Can you work these out from the model? Positions are in its coordinate system, mm. A direction names the side the tool comes from. Give positions to 0.01 mm unless a question says otherwise; leave off trailing zeros. Order: outer loops, then holes, each group sorted by start corner. A loop starts at its lowest first (then second) coordinate and runs counter-clockwise, first axis right, second up. Notation, with made-up numbers: (59, 72) - (74, 72) arc R24 ccw to (74, 109) - close; hole circle Ø9 at (50.25, 35.25). An arc over 180 degrees is marked (long way). Use one line per item in the form item = value. Start each with the question number.
1) Suppose I cut it at B-B, the plane z = 2. Write out the boundary of the cut face in (x, y).
2) Please list where these lines run through material, in increasing order: probe 1 along X at (y, z) = (0, -3); probe 2 along Y at (x, z) = (0, 0); probe 3 along Y at (x, z) = (2.35, -5).
3) We'd pull the mould along Z, two halves only. Please class faces 1 (the flat face through (-3, 0, 9.4)), 2 (the cylindrical face through (2.88, 0.08, -6.75)), 3 (the flat face through (5, 0, 0.2)): released by +Z, released by -Z, zero draft, split by the parting line, or undercut.
4) For pin 1 (4 mm diameter, centred on x = -1.5, z = -0.5, fed in from +Y); pin 2 (0.9 mm diameter, centred on y = -0.5, z = 1, fed in from -X); pin 3 (1.5 mm diameter, centred on x = -5, z = 7, fed in from -Y), each with a flat end and sliding along its axis, tell me the tip position at first contact or that it passes through.
5) Which directions (+Z, -Z, +X, -X, +Y, -Y) give clear straight access to the entire face, cutting with the end or side of a thin tool? Please do faces 4 (the flat face through (2, 3.65, -4)), 5 (the cylindrical face through (-4.794, 0.264, 2.572)), 6 (the flat face through (2, 0, -8)), 7 (the flat face through (2, -3.65, -4)), 8 (the cylindrical face through (-3.65, 0.08, -4.24)).
6) Suppose I cut it at A-A, the plane z = -5. Write out the boundary of the cut face in (x, y), and give its area (3 significant figures).
```python
from build123d import *

# Parameters (mm, degrees)
BOSS_EXTRUDE4_DEPTH            = 4.2
BOSS_EXTRUDE4_DEPTH_BACK       = 0.2
SKETCH10_R                     = 6
BOSS_EXTRUDE5_DEPTH            = 9
SKETCH16_R                     = 6
BOSS_EXTRUDE6_DEPTH            = 4.8
CUT_EXTRUDE2_DEPTH             = 21.471443525
F_3_5_3_5_DIAMETER_HOLE0_D     = 3.5
F_3_5_3_5_DIAMETER_HOLE0_DEPTH = 4
F_3_5_3_5_DIAMETER_HOLE0_TIP   = 1.051506083
CHAMFER2_SIZE                  = 0.4


with BuildPart() as part:
    # Sketch10 → Boss-Extrude4 (new, two sides: drawn at the far end of the back side and taken through both)
    with BuildSketch(Plane.XY.offset(0.4).offset(-BOSS_EXTRUDE4_DEPTH_BACK)):
        with Locations((1.2, 0)):
            Circle(SKETCH10_R)
    extrude(amount=BOSS_EXTRUDE4_DEPTH + BOSS_EXTRUDE4_DEPTH_BACK)

    # Sketch11 → Boss-Extrude5 (add)
    with BuildSketch(Plane(origin=(0, 0, 0.2), x_dir=(-1, 0, 0), z_dir=(0, 0, -1))):
        with BuildLine():
            Line((-4, -3.05), (-4, 3.05))
            ThreePointArc((-4, 3.05), (-3.824264069, 3.474264069), (-3.4, 3.65))
            Line((-3.4, 3.65), (0, 3.65))
            ThreePointArc((0, 3.65), (3.65, 0), (0, -3.65))
            Line((0, -3.65), (-3.4, -3.65))
            ThreePointArc((-3.4, -3.65), (-3.824264069, -3.474264069), (-4, -3.05))
        make_face()
    extrude(amount=BOSS_EXTRUDE5_DEPTH)

    # Sketch16 → Boss-Extrude6 (add)
    with BuildSketch(Plane(origin=(0, 0, 4.6), x_dir=(-1, 0, 0), z_dir=(0, 0, -1))):
        with Locations((1, 0)):
            Circle(SKETCH16_R)
    extrude(amount=-BOSS_EXTRUDE6_DEPTH)

    # Sketch17 → Cut-Extrude2 (cut, through all)
    with BuildSketch(Plane.XY.offset(9.4)):
        with BuildLine():
            Line((2, -1.5), (2, 1.5))
            ThreePointArc((2, 1.5), (-2.5, 0), (2, -1.5))
        make_face()
    extrude(amount=-CUT_EXTRUDE2_DEPTH, mode=Mode.SUBTRACT)

    # Ø3.5 (3.5) Diameter Hole0
    with Locations(Plane(origin=(4, 0, 0), x_dir=(0, 0, -1), z_dir=(1, 0, 0))):
        with Locations((5, 0)):
            Hole(F_3_5_3_5_DIAMETER_HOLE0_D / 2, depth=F_3_5_3_5_DIAMETER_HOLE0_DEPTH)
            with Locations((0, 0, -(F_3_5_3_5_DIAMETER_HOLE0_DEPTH + F_3_5_3_5_DIAMETER_HOLE0_TIP / 2))):  # 118° drill point
                Cone(0, F_3_5_3_5_DIAMETER_HOLE0_D / 2, F_3_5_3_5_DIAMETER_HOLE0_TIP, mode=Mode.SUBTRACT)

    # Chamfer2
    chamfer2_edges = [part.edges().sort_by_distance(p)[0] for p in [
        (5, 0, 9.4),
        (-4.8, 0, 0.2),
    ]]
    chamfer(chamfer2_edges, length=CHAMFER2_SIZE)


solid = part.part
```
Result sheet:
q1.outline = circle Ø12 at (1.2, 0); hole (2, -1.5) - (2, 1.5) arc R2.5 ccw (long way) to start
q2.probe_1 = -3.65 to -2.5, 2 to 4
q2.probe_2 = -3.65 to -2.5, 2.5 to 3.65
q2.probe_3 = -3.65 to -1.75, 1.75 to 3.65
q3.face_1 = released by +Z
q3.face_2 = undercut
q3.face_3 = released by -Z
q4.pin_1 = 5.91
q4.pin_2 = -4.8
q4.pin_3 = -5.04
q5.face_4 = -Z, +X, -X, +Y
q5.face_5 = -Z
q5.face_6 = +Z, -Z
q5.face_7 = -Z, +X, -X, -Y
q5.face_8 = -Z, -X
q6.outline = (0, -3.65) - (3.4, -3.65) arc R0.6 ccw to (4, -3.05) - (4, -1.75) - (1.79, -1.75) arc R2.5 cw (long way) to (1.79, 1.75) - (4, 1.75) - (4, 3.05) arc R0.6 ccw to (3.4, 3.65) - (0, 3.65) arc R3.65 ccw to start
q6.area = 24.3 mm²
